Answer from the drawing. Dimensions are ordinates in mm from the lowest x, y and z of the part. A direction names the side the tool comes from. Coordinates: 2 decimals unless noted, no trailing zeros. Loops run counter-clockwise (first coordinate to the right, second up) from the corner with the lowest first, then second, coordinate; pieces in that order, holes last.
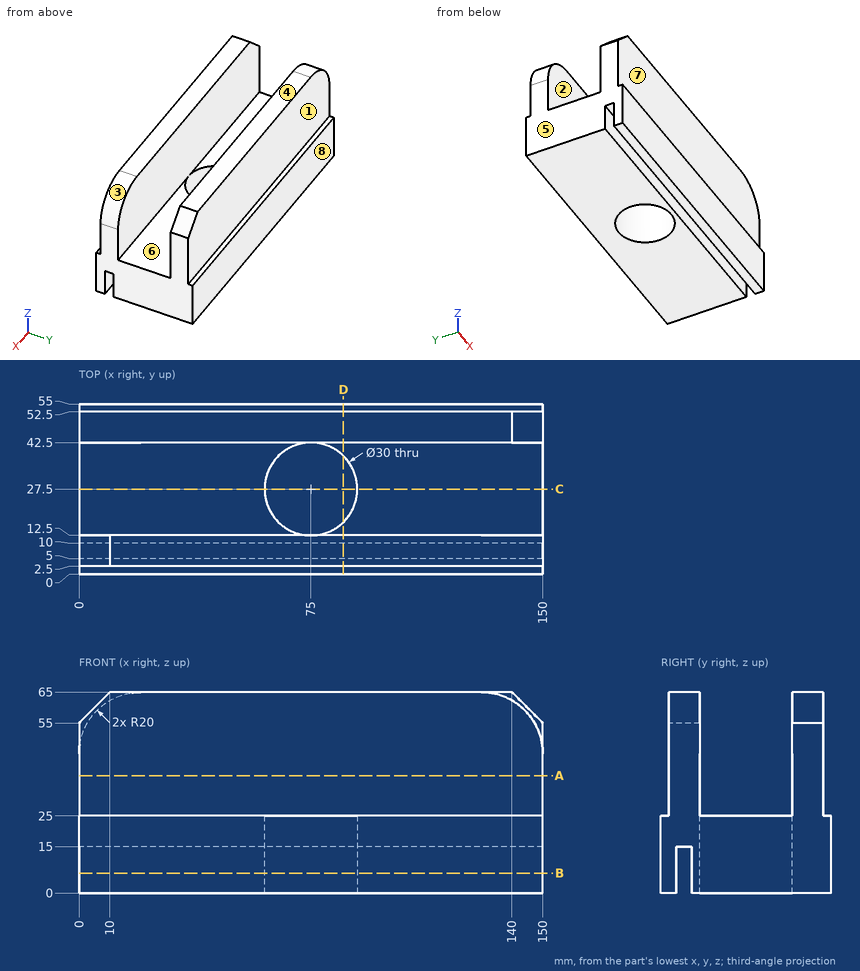
Item 1: A cutting plane is placed at B-B on z = 6.5. Determine the outline of the cut face in (x, y), then the cut area to 3 significant figures.
Numbers:
outline: (0, 0) - (150, 0) - (150, 5) - (0, 5) - close; (0, 10) - (150, 10) - (150, 55) - (0, 55) - close; hole circle Ø30 at (75, 27.5)
area: 6,790 mm2
Item 2: Find the intervals of material crossed by line 1 along Y through (x, z) = (75, 8.5); line 2 along Y through (x, z) = (76, 44.5); line 3 along X through (y, z) = (27.5, 5), in increasing order.
Numbers:
line 1: y = 0 to 5, 10 to 12.5, 42.5 to 55
line 2: y = 2.5 to 12.5, 42.5 to 52.5
line 3: x = 0 to 60, 90 to 150
Item 3: A cutting plane is placed at A-A on z = 38. Determine the outline of the cut face in (x, y), then the cut area to 3 significant figures.
Numbers:
outline: (0, 2.5) - (150, 2.5) - (150, 12.5) - (0, 12.5) - close; (0, 42.5) - (150, 42.5) - (150, 52.5) - (0, 52.5) - close
area: 3,000 mm2
Item 4: A cutting plane is placed at D-D on x = 85.5. Determine the outline of the cut face in (y, z), then the cut area to 3 significant figures.
Numbers:
outline: (0, 0) - (5, 0) - (5, 15) - (10, 15) - (10, 0) - (16.79, 0) - (16.79, 25) - (12.5, 25) - (12.5, 65) - (2.5, 65) - (2.5, 25) - (0, 25) - close; (38.21, 0) - (55, 0) - (55, 25) - (52.5, 25) - (52.5, 65) - (42.5, 65) - (42.5, 25) - (38.21, 25) - close
area: 1,560 mm2
Item 5: Which of the six approach directions +Z, -Z, +X, -X, +Y, -Y give full straight-line access (tool end or side, diameter ignored) to the marked faces 1, 2, 3 and 4?
Numbers:
face 1: +Z, +X, -X, +Y
face 2: +Z, +X, -X
face 3: +Z, +X, -Y
face 4: +Z, +X, -X, +Y, -Y
Item 6: A cutting plane is placed at C-C on y = 27.5. Determine the outline of the cut face in (x, z), then the cut area to 3 significant figures.
Numbers:
outline: (0, 0) - (60, 0) - (60, 25) - (0, 25) - close; (90, 0) - (150, 0) - (150, 25) - (90, 25) - close
area: 3,000 mm2
Item 7: Determine the mould class of the marked faces 5, 6, 7 and 8 for opening direction Y: released by +Y, released by -Y, zero draft, split by the parting line, or undercut.
Numbers:
face 5: zero draft
face 6: undercut
face 7: released by -Y
face 8: released by +Y
Item 8: Given pin 1 (5 mm diameter, centred on y = 14.5, z = 29, fed in from -X); pin 2 (1.5 mm diameter, centred on x = 35, y = 33, fed in from +Z); pin 3 (12 mm diameter, centred on x = 40, z = 37, fed in from -Y); pin 4 (12 mm diameter, centred on x = 112, z = 50.5, fed in from +Y), each flat-ended and moving along its own axis, determine where each tip first touches the part or whether it passes through.
Numbers:
pin 1: stops at x = 0
pin 2: stops at z = 25
pin 3: stops at y = 2.5
pin 4: stops at y = 52.5
